Model file for the job. Use its own axes, mm. A direction names the side the tool comes from. Give positions to 0.01 mm unless a question says otherwise; leave off trailing zeros. Order: outer loops, then holes, each group sorted by start corner. A loop starts at its lowest first (then second) coordinate and runs counter-clockwise, first axis right, second up. Notation, with made-up numbers: (0, -6) -> (11, -6) arc R25 ccw to (11, 9) -> close; hole circle Ø9 at (44.25, 17.5). An arc over 180 degrees is marked (long way). Use CSV: the item, a comma, the result in double quotes. Start each with the question number.
1. Cut at C-C on y = 5.5. List the corners of the cut face in (x, z).
2. Pull direction Y, two halves, no side cores. Call faces 1 (the flat face through (163, 14, 11)), 2 (the flat face through (91, -10, 26)), 3 (the flat face through (106, 21.1, 13)): released by +Y, released by -Y, zero draft, split by the parting line, or undercut.
3. Wall check: line 1 (Y direction, x = 137.15, z = 9.6); line 2 (Y direction, x = 163.5, z = 9.2); line 3 (Y direction, x = 207, z = 1.75). Give the ranges that are in metal, low to high. Write a range as from..to.
4. 3-axis set-ups, long thin cutter, end or side, ignore diameter. For faces 4 (the cylindrical face through (139.058, 14.801, 8.465)), 5 (the flat face through (106, 12, 0)), 6 (the flat face through (219, 6, 16.5)): which of +Z, -Z, +X, -X, +Y, -Y reach the whole face in a straight line?
5. Cut at A-A on x = 88. List the corners of the cut face in (y, z).
6. Cut at B-B on z = 23.5. List the corners of the cut face in (x, y).
7. Drop flat-ended pins along their axis: pin 1 (1.2 mm diameter, centred on x = 163, y = -6, fed in from +Z); pin 2 (2.5 mm diameter, centred on x = 1.5, y = 3.5, fed in from -Z); pin 3 (7.5 mm diameter, centred on x = 65, y = 12.5, fed in from +Z). Give the stop position or say it passes through.
```python
from build123d import *

# Parameters (mm, degrees)
SKETCH_1_W          = 226
SKETCH_1_H          = 34
SKETCH_1_W_2        = 216
SKETCH_1_H_2        = 8.2
EXTRUDE_1_DEPTH     = 6
SKETCH_2_R          = 2
EXTRUDE_2_DEPTH     = 5
SKETCH_3_R          = 0.75
CUT_EXTRUDE_1_DEPTH = 5
SKETCH_4_W          = 226
SKETCH_4_H          = 34
SKETCH_4_W_2        = 210
SKETCH_4_H_2        = 27
EXTRUDE_3_DEPTH     = 2
SKETCH_6_W          = 226
SKETCH_6_H          = 34
SKETCH_6_W_2        = 214.5
SKETCH_6_H_2        = 27
EXTRUDE_4_DEPTH     = 18
SKETCH_7_W          = 1.5
SKETCH_7_H          = 27
CUT_EXTRUDE_2_DEPTH = 2
SKETCH_8_R          = 2
EXTRUDE_5_DEPTH     = 5
SKETCH_9_R          = 0.75
CUT_EXTRUDE_3_DEPTH = 5
SKETCH_10_W         = 4
SKETCH_10_H         = 10
CUT_EXTRUDE_4_DEPTH = 5


with BuildPart() as part:
    # Эскиз1 → Бобышка-Вытянуть1 (new body)
    with BuildSketch(Plane.XY):
        with Locations((108, 4.1)):
            Rectangle(SKETCH_1_W, SKETCH_1_H)
        with Locations((108, 4.1)):
            Rectangle(SKETCH_1_W_2, SKETCH_1_H_2, mode=Mode.SUBTRACT)
    extrude(amount=EXTRUDE_1_DEPTH)

    # Эскиз2 → Бобышка-Вытянуть2 (add)
    with BuildSketch(Plane.XY.offset(6)):
        with Locations((78.85, 14.2)):
            Circle(SKETCH_2_R)
        with Locations((78.85, -6)):
            Circle(SKETCH_2_R)
        with Locations((137.15, 14.2)):
            Circle(SKETCH_2_R)
        with Locations((137.15, -6)):
            Circle(SKETCH_2_R)
    extrude(amount=EXTRUDE_2_DEPTH)

    # Эскиз3 → Вырез-Вытянуть1 (cut)
    with BuildSketch(Plane.XY.offset(11)):
        with Locations((78.85, 14.2)):
            Circle(SKETCH_3_R)
        with Locations((78.85, -6)):
            Circle(SKETCH_3_R)
        with Locations((137.15, 14.2)):
            Circle(SKETCH_3_R)
        with Locations((137.15, -6)):
            Circle(SKETCH_3_R)
    extrude(amount=-CUT_EXTRUDE_1_DEPTH, mode=Mode.SUBTRACT)

    # Эскиз4 → Бобышка-Вытянуть3 (add)
    with BuildSketch(Plane.XY.offset(6)):
        with Locations((108, 4.1)):
            Rectangle(SKETCH_4_W, SKETCH_4_H)
        with Locations((108, 4.1)):
            Rectangle(SKETCH_4_W_2, SKETCH_4_H_2, mode=Mode.SUBTRACT)
    extrude(amount=EXTRUDE_3_DEPTH)

    # Эскиз6 → Бобышка-Вытянуть4 (add)
    with BuildSketch(Plane.XY.offset(8)):
        with Locations((108, 4.1)):
            Rectangle(SKETCH_6_W, SKETCH_6_H)
        with Locations((110.25, 4.1)):
            Rectangle(SKETCH_6_W_2, SKETCH_6_H_2, mode=Mode.SUBTRACT)
    extrude(amount=EXTRUDE_4_DEPTH)

    # Эскиз7 → Вырез-Вытянуть2 (cut)
    with BuildSketch(Plane.ZY.offset(-217.5)):
        with Locations((11.75, 4.1)):
            Rectangle(SKETCH_7_W, SKETCH_7_H)
    extrude(amount=-CUT_EXTRUDE_2_DEPTH, mode=Mode.SUBTRACT)

    # Эскиз8 → Бобышка-Вытянуть5 (add)
    with BuildSketch(Plane.XY.offset(6)):
        with Locations((163.5, 14.85)):
            Circle(SKETCH_8_R)
        with Locations((163.5, -6.65)):
            Circle(SKETCH_8_R)
    extrude(amount=EXTRUDE_5_DEPTH)

    # Эскиз9 → Вырез-Вытянуть3 (cut)
    with BuildSketch(Plane.XY.offset(11)):
        with Locations((163.5, 14.85)):
            Circle(SKETCH_9_R)
        with Locations((163.5, -6.65)):
            Circle(SKETCH_9_R)
    extrude(amount=-CUT_EXTRUDE_3_DEPTH, mode=Mode.SUBTRACT)

    # Эскиз10 → Вырез-Вытянуть4 (cut)
    with BuildSketch(Plane.ZY.offset(-217.5)):
        with Locations((14.5, 6.1)):
            Rectangle(SKETCH_10_W, SKETCH_10_H)
    extrude(amount=-CUT_EXTRUDE_4_DEPTH, mode=Mode.SUBTRACT)


solid = part.part
```
Verdict:
1,outline,"(-5, 0) -> (0, 0) -> (0, 6) -> (3, 6) -> (3, 26) -> (-5, 26) -> close; (213, 6) -> (216, 6) -> (216, 0) -> (221, 0) -> (221, 12.5) -> (219.5, 12.5) -> (219.5, 11) -> (217.5, 11) -> (217.5, 8) -> (213, 8) -> close; (217.5, 16.5) -> (221, 16.5) -> (221, 26) -> (217.5, 26) -> close"
2,face 1,"undercut"
2,face 2,"zero draft"
2,face 3,"released by +Y"
3,line 1,"-12.9..-9.4, -8..-6.75, -5.25..-4, 12.2..13.45, 14.95..16.2, 17.6..21.1"
3,line 2,"-12.9..-9.4, -8.65..-7.4, -5.9..-4.65, 12.85..14.1, 15.6..16.85, 17.6..21.1"
3,line 3,"-12.9..0, 8.2..21.1"
4,face 4,"+Z"
4,face 5,"-Z, +X, -X, +Y, -Y"
4,face 6,"+X"
5,outline,"(-12.9, 0) -> (0, 0) -> (0, 6) -> (-9.4, 6) -> (-9.4, 26) -> (-12.9, 26) -> close; (8.2, 0) -> (21.1, 0) -> (21.1, 26) -> (17.6, 26) -> (17.6, 6) -> (8.2, 6) -> close"
6,outline,"(-5, -12.9) -> (221, -12.9) -> (221, 21.1) -> (-5, 21.1) -> close; hole (3, -9.4) -> (217.5, -9.4) -> (217.5, 17.6) -> (3, 17.6) -> close"
7,pin 1,"z = 11"
7,pin 2,"z = 6"
7,pin 3,"z = 6"
